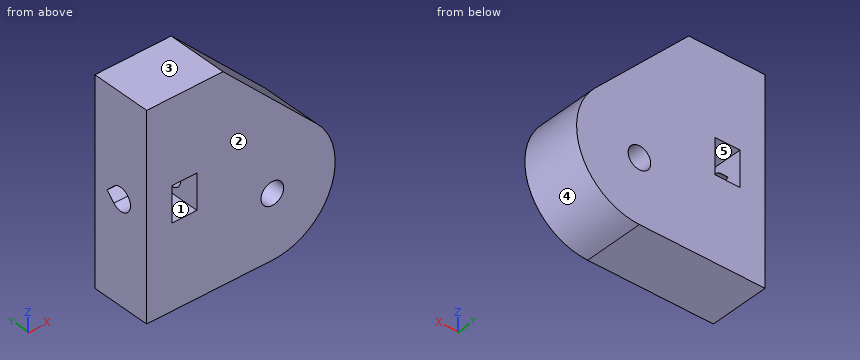
from build123d import *

# Parameters (mm, degrees)
SKETCH1_R           = 2.25
BOSS_EXTRUDE1_DEPTH = 12
CUT_EXTRUDE1_DEPTH  = 20
CUT_EXTRUDE2_REACH  = 41.054
SKETCH3_W           = 5
SKETCH3_H           = 7


with BuildPart() as part:
    # Sketch1 → Boss-Extrude1 (new body)
    with BuildSketch(Plane(origin=(0, 0, 0), x_dir=(1, 0, 0), z_dir=(0, 1, 0))):
        with BuildLine():
            Line((0, 12.5), (-15, 12.5))
            Line((-15, 12.5), (-25, 12.5))
            Line((-25, 12.5), (-25, -27.5))
            Line((-25, -27.5), (-9.82233047, -27.5))
            Line((-9.82233047, -27.5), (8.838834765, -8.838834765))
            ThreePointArc((8.838834765, -8.838834765), (11.548494156, 4.783542905), (0, 12.5))
        make_face()
        with Locations(Location((0, 0, 0), (0, 0, 270))):
            Circle(SKETCH1_R, mode=Mode.SUBTRACT)
    extrude(amount=BOSS_EXTRUDE1_DEPTH)

    # Sketch2 → Cut-Extrude1 (cut)
    with BuildSketch(Plane.ZY.offset(25)):
        with BuildLine():
            Line((5.909009742, 7.590990258), (7.5, 9.181980515))
            Line((7.5, 9.181980515), (9.090990258, 7.590990258))
            ThreePointArc((9.090990258, 7.590990258), (7.5, 3.75), (5.909009742, 7.590990258))
        make_face()
    extrude(amount=-CUT_EXTRUDE1_DEPTH, mode=Mode.SUBTRACT)

    # Sketch3 → Cut-Extrude2 (cut, up to next)
    with BuildSketch(Plane(origin=(0, 12, 0), x_dir=(1, 0, 0), z_dir=(0, 1, 0)), mode=Mode.PRIVATE) as cut_extrude2_sk1:
        with Locations((-17.5, -7.5)):
            Rectangle(SKETCH3_W, SKETCH3_H)
    cut_extrude2_tool1 = extrude(cut_extrude2_sk1.sketch, amount=-CUT_EXTRUDE2_REACH, mode=Mode.PRIVATE) & part.part
    add(cut_extrude2_tool1.solids().sort_by_distance((-17.5, 12, 7.5))[0], mode=Mode.SUBTRACT)


solid = part.part
Geometry: final body of the model. Coordinates: model frame, mm. Face numbers are marked on the shaded views. A direction names the side the tool comes from. Round coordinates to 2 decimals unless told otherwise and drop trailing zeros. Order: outer loops, then holes, each group sorted by start corner. A loop starts at its lowest first (then second) coordinate and runs counter-clockwise, first axis right, second up.
Q1. Access query for the marked faces 1 and 2. Directions: +Z, -Z, +X, -X, +Y, -Y. A direction counts if a zero-diameter tool reaches every point of the face in a straight line with its end or side. Return the directions, or none.
Result sheet:
face 1: +Y, -Y
face 2: +Z, -Z, +X, -X, -Y
Q2. Section C-C, the plane x = -14. Output: boundary loops of the cut face in (y, z).
Result sheet:
outline: (0, -12.5) - (12, -12.5) - (12, 27.5) - (0, 27.5) - close; hole (7.59, 5.91) - (9.18, 7.5) - (7.59, 9.09) arc R2.25 ccw (long way) to start
Q3. Mould query, pull axis Z, two halves, no side actions, for the marked faces 3, 4 and 5. Classes: released by +Z, released by -Z, zero draft, split by the parting line, or undercut.
Result sheet:
face 3: released by +Z
face 4: split by the parting line
face 5: undercut
Q4. Section B-B, the plane z = 0. Output: boundary loops of the cut face in (x, y), and give its area (3 significant figures).
Result sheet:
outline: (-25, 0) - (-2.25, 0) - (-2.25, 12) - (-25, 12) - close; (2.25, 0) - (12.5, 0) - (12.5, 12) - (2.25, 12) - close
area: 396 mm2
Q5. Pin query (flat end, axial travel): pin 1 (1.4 mm diameter, centred on y = 5.5, z = 8, fed in from -X); pin 2 (7 mm diameter, centred on x = 0, z = 0, fed in from -Y); pin 3 (1 mm diameter, centred on x = -3.5, y = 4.5, fed in from +Z); pin 4 (6 mm diameter, centred on x = 5, y = 3.5, fed in from -Z). Return the tip coordinate at first contact, or that it passes through.
Result sheet:
pin 1: stops at x = -5
pin 2: stops at y = 0
pin 3: stops at z = 21.68
pin 4: stops at z = -12.34
Q6. Material intervals for probe 1 along Z at (x, y) = (-21.6, 6); probe 2 along Z at (x, y) = (-19.5, 11); probe 3 along X at (y, z) = (3.5, 0), sorted ascending.
Result sheet:
probe 1: z = -12.5 to 5.25, 9.75 to 27.5
probe 2: z = -12.5 to 4, 11 to 27.5
probe 3: x = -25 to -2.25, 2.25 to 12.5
Q7. Section D-D, the plane y = 6. Output: boundary loops of the cut face in (x, z).
Result sheet:
outline: (-25, -12.5) - (0, -12.5) arc R12.5 ccw to (8.84, 8.84) - (-9.82, 27.5) - (-25, 27.5) - (-25, 9.75) - (-20, 9.75) - (-20, 11) - (-15, 11) - (-15, 9.75) - (-5, 9.75) - (-5, 5.25) - (-15, 5.25) - (-15, 4) - (-20, 4) - (-20, 5.25) - (-25, 5.25) - close; hole circle Ø4.5 at (0, 0)
Q8. Section A-A, the plane y = 2.5. Output: boundary loops of the cut face in (x, z), and give its area (3 significant figures).
Result sheet:
outline: (-25, -12.5) - (0, -12.5) arc R12.5 ccw to (8.84, 8.84) - (-9.82, 27.5) - (-25, 27.5) - close; hole (-20, 4) - (-15, 4) - (-15, 11) - (-20, 11) - close; hole circle Ø4.5 at (0, 0)
area: 1,160 mm2
